For this review, take the finished solid that the model builds, in its own axes (mm). A direction names the side the tool comes from. Round coordinates to 2 decimals unless told otherwise and drop trailing zeros. Order: outer loops, then holes, each group sorted by start corner. A loop starts at its lowest first (then second) coordinate and runs counter-clockwise, first axis right, second up. Notation, with made-up numbers: M 11,32.5 L 42,32.5 A23 cw 42,56.5 Z; hole C 80.25,77 d6. An arc over 180 degrees is marked long. Use a Markdown table: item, result.
from build123d import *

# Parameters (mm, degrees)
SKETCH2_W            = 59
SKETCH2_H            = 39.64
BOSS_EXTRUDE1_DEPTH  = 2
BOSS_EXTRUDE2_DEPTH  = 87.25
SKETCH4_W            = 59
SKETCH4_H            = 39.64
BOSS_EXTRUDE4_DEPTH  = 2
BOSS_EXTRUDE5_DEPTH  = 59
SKETCH5_3_W          = 2
SKETCH5_3_H          = 10
BOSS_EXTRUDE6_DEPTH  = 59
BOSS_EXTRUDE7_DEPTH  = 59
BOSS_EXTRUDE8_DEPTH  = 6
SKETCH8_W            = 38.6
SKETCH8_H            = 87.25
CUT_EXTRUDE1_DEPTH   = 12.5
SKETCH9_W            = 15.5
SKETCH9_H            = 10.65
CUT_EXTRUDE2_DEPTH   = 13.6
SKETCH9_4_W          = 21.1
SKETCH9_4_H          = 7.5
CUT_EXTRUDE3_DEPTH   = 8.6
SKETCH10_W           = 67.65
SKETCH10_H           = 14.625
BOSS_EXTRUDE9_DEPTH  = 7.9
BOSS_EXTRUDE10_DEPTH = 4
SKETCH11_W           = 25
SKETCH11_H           = 7.9
BOSS_EXTRUDE14_DEPTH = 22
SKETCH12_W           = 25
SKETCH12_H           = 10
CUT_EXTRUDE4_DEPTH   = 3.9


with BuildPart() as part:
    # Sketch2 → Boss-Extrude1 (new body)
    with BuildSketch(Plane.XY):
        Polygon((-256.9, 47.64), (-256.9, 0), (0, 0), (0, 41.64), (-2, 41.64), (-2, 9.9), (-8.85, 9.9), (-8.85, 2), (-144.15, 2), (-144.15, 9.9), (-151, 9.9), (-151, 41.64), (-153, 41.64), (-191.6, 41.64), (-193.6, 41.64), (-193.6, 2), (-252.6, 2), (-252.6, 41.64), (-254.9, 41.64), (-254.9, 45.64), (-252.6, 45.64), (-252.6, 47.64), align=None)
        with Locations((-223.1, 21.82)):
            Rectangle(SKETCH2_W, SKETCH2_H)
        Polygon((-151, 41.64), (-2, 41.64), (-2, 9.9), (-8.85, 9.9), (-8.85, 2), (-144.15, 2), (-144.15, 9.9), (-151, 9.9), align=None)
    extrude(amount=-BOSS_EXTRUDE1_DEPTH)

    # Sketch2_3 → Boss-Extrude2 (add)
    with BuildSketch(Plane.XY):
        Polygon((-256.9, 47.64), (-256.9, 0), (0, 0), (0, 41.64), (-2, 41.64), (-2, 9.9), (-8.85, 9.9), (-8.85, 2), (-144.15, 2), (-144.15, 9.9), (-151, 9.9), (-151, 41.64), (-153, 41.64), (-191.6, 41.64), (-193.6, 41.64), (-193.6, 2), (-252.6, 2), (-252.6, 41.64), (-254.9, 41.64), (-254.9, 45.64), (-252.6, 45.64), (-252.6, 47.64), align=None)
    extrude(amount=BOSS_EXTRUDE2_DEPTH)

    # Sketch4 → Boss-Extrude4 (add)
    with BuildSketch(Plane.XY.offset(87.25)):
        Polygon((-256.9, 47.64), (-256.9, 41.64), (-254.9, 41.64), (-254.9, 45.64), (-252.6, 45.64), (-252.6, 47.64), align=None)
        with Locations((-223.1, 21.82)):
            Rectangle(SKETCH4_W, SKETCH4_H)
        Polygon((-254.9, 41.64), (-256.9, 41.64), (-256.9, 0), (0, 0), (0, 41.64), (-2, 41.64), (-2, 9.9), (-8.85, 9.9), (-8.85, 2), (-144.15, 2), (-144.15, 9.9), (-151, 9.9), (-151, 41.64), (-193.6, 41.64), (-193.6, 2), (-252.6, 2), (-252.6, 41.64), align=None)
        Polygon((-2, 41.64), (-151, 41.64), (-151, 9.9), (-144.15, 9.9), (-144.15, 2), (-8.85, 2), (-8.85, 9.9), (-2, 9.9), align=None)
    extrude(amount=BOSS_EXTRUDE4_DEPTH)

    # Sketch5 → Boss-Extrude5 (add)
    with BuildSketch(Plane(origin=(-252.6, 0, 0), x_dir=(0, 0, -1), z_dir=(1, 0, 0))):
        Polygon((-72.69, 2), (-40.014243309, 31.64), (-42.014243309, 31.64), (-56.208170838, 18.764766047), (-87.25, 18.764766047), (-87.25, 2), align=None)
        Polygon((0, 2), (0, 31.64), (-10, 31.64), (-21.014243309, 31.64), (-53.69, 2), align=None)
    extrude(amount=BOSS_EXTRUDE5_DEPTH)

    # Sketch5_3 → Boss-Extrude6 (add)
    with BuildSketch(Plane(origin=(-252.6, 0, 0), x_dir=(0, 0, -1), z_dir=(1, 0, 0))):
        with Locations((-41.014243309, 36.64)):
            Rectangle(SKETCH5_3_W, SKETCH5_3_H)
    extrude(amount=BOSS_EXTRUDE6_DEPTH)

    # Sketch6 → Boss-Extrude7 (add)
    with BuildSketch(Plane(origin=(-252.6, 0, 0), x_dir=(0, 0, -1), z_dir=(1, 0, 0))):
        with BuildLine():
            Line((-42.014243309, 31.64), (-42.014243309, 41.64))
            ThreePointArc((-42.014243309, 41.64), (-48.969941413, 25.441110515), (-65.285951379, 18.764766047))
            Line((-65.285951379, 18.764766047), (-56.208170838, 18.764766047))
            Line((-56.208170838, 18.764766047), (-42.014243309, 31.64))
        make_face()
    extrude(amount=BOSS_EXTRUDE7_DEPTH)

    # Sketch7 → Boss-Extrude8 (add)
    with BuildSketch(Plane(origin=(0, 41.64, 0), x_dir=(1, 0, 0), z_dir=(0, 1, 0))):
        Polygon((0, -89.25), (0, 2), (-254.9, 2), (-254.9, 0), (-252.6, 0), (-2, 0), (-2, -87.25), (-252.6, -87.25), (-254.9, -87.25), (-254.9, -89.25), align=None)
    extrude(amount=BOSS_EXTRUDE8_DEPTH)

    # Sketch8 → Cut-Extrude1 (cut)
    with BuildSketch(Plane(origin=(0, 41.64, 0), x_dir=(1, 0, 0), z_dir=(0, 1, 0))):
        with Locations((-172.3, -43.625)):
            Rectangle(SKETCH8_W, SKETCH8_H)
    extrude(amount=-CUT_EXTRUDE1_DEPTH, mode=Mode.SUBTRACT)

    # Sketch9 → Cut-Extrude2 (cut)
    with BuildSketch(Plane(origin=(0, 29.14, 0), x_dir=(1, 0, 0), z_dir=(0, 1, 0))):
        with Locations((-160.75, -16.325)):
            Rectangle(SKETCH9_W, SKETCH9_H)
        with Locations((-183.85, -29.975)):
            Rectangle(SKETCH9_W, SKETCH9_H)
        with Locations((-160.75, -43.625)):
            Rectangle(SKETCH9_W, SKETCH9_H)
        with Locations((-183.85, -57.275)):
            Rectangle(SKETCH9_W, SKETCH9_H)
        with Locations((-160.75, -70.925)):
            Rectangle(SKETCH9_W, SKETCH9_H)
    extrude(amount=-CUT_EXTRUDE2_DEPTH, mode=Mode.SUBTRACT)

    # Sketch9_4 → Cut-Extrude3 (cut)
    with BuildSketch(Plane(origin=(0, 29.14, 0), x_dir=(1, 0, 0), z_dir=(0, 1, 0))):
        with Locations((-181.05, -16.325)):
            Rectangle(SKETCH9_4_W, SKETCH9_4_H)
        with Locations((-163.55, -29.975)):
            Rectangle(SKETCH9_4_W, SKETCH9_4_H)
        with Locations((-181.05, -43.625)):
            Rectangle(SKETCH9_4_W, SKETCH9_4_H)
        with Locations((-163.55, -57.275)):
            Rectangle(SKETCH9_4_W, SKETCH9_4_H)
        with Locations((-181.05, -70.925)):
            Rectangle(SKETCH9_4_W, SKETCH9_4_H)
    extrude(amount=-CUT_EXTRUDE3_DEPTH, mode=Mode.SUBTRACT)

    # Sketch10 → Boss-Extrude9 (add)
    with BuildSketch(Plane(origin=(0, 2, 0), x_dir=(1, 0, 0), z_dir=(0, 1, 0))):
        with Locations((-110.325, -7.3125)):
            Rectangle(SKETCH10_W, SKETCH10_H)
        with Locations((-42.675, -7.3125)):
            Rectangle(SKETCH10_W, SKETCH10_H)
        with Locations((-42.675, -79.9375)):
            Rectangle(SKETCH10_W, SKETCH10_H)
        with Locations((-110.325, -79.9375)):
            Rectangle(SKETCH10_W, SKETCH10_H)
    extrude(amount=BOSS_EXTRUDE9_DEPTH)

    # Sketch10_4 → Boss-Extrude10 (add)
    with BuildSketch(Plane(origin=(0, 2, 0), x_dir=(1, 0, 0), z_dir=(0, 1, 0))):
        Polygon((-8.85, -36.625), (-144.15, -36.625), (-144.15, -72.625), (-76.5, -72.625), (-8.85, -72.625), align=None)
    extrude(amount=BOSS_EXTRUDE10_DEPTH)

    # Sketch11 → Boss-Extrude14 (add)
    with BuildSketch(Plane.XY.offset(14.625)):
        with Locations((-131.65, 5.95)):
            Rectangle(SKETCH11_W, SKETCH11_H)
        with Locations((-21.35, 5.95)):
            Rectangle(SKETCH11_W, SKETCH11_H)
    extrude(amount=BOSS_EXTRUDE14_DEPTH)

    # Sketch12 → Cut-Extrude4 (cut)
    with BuildSketch(Plane(origin=(0, 9.9, 0), x_dir=(1, 0, 0), z_dir=(0, 1, 0))):
        with Locations((-131.65, -31.625)):
            Rectangle(SKETCH12_W, SKETCH12_H)
        with Locations((-21.35, -31.625)):
            Rectangle(SKETCH12_W, SKETCH12_H)
    extrude(amount=-CUT_EXTRUDE4_DEPTH, mode=Mode.SUBTRACT)


solid = part.part
Q1. Add section C-C (y = 38). Write out the cut boundary in (x, z).
Determined:
| item | result |
|---|---|
| outline | M -256.9,-2 L 0,-2 L 0,89.25 L -256.9,89.25 Z; hole M -252.6,0 L -193.6,0 L -193.6,40.01 L -252.6,40.01 Z; hole M -252.6,42.36 L -193.6,42.36 L -193.6,87.25 L -252.6,87.25 Z; hole M -191.6,0 L -153,0 L -153,87.25 L -191.6,87.25 Z; hole M -151,0 L -2,0 L -2,87.25 L -151,87.25 Z |
Q2. Wall thickness on line 1 along X through (y, z) = (31, 25.5); line 2 along Z through (x, y) = (-172, 26) (3 decimals); line 3 along X through (y, z) = (9, 49.5): over which ranges is each line inside the solid? List them lowest first. Write a range as [from, to].
Determined:
| item | result |
|---|---|
| line 1 | x = [-256.9, -252.6], [-193.6, -191.6], [-153, -151], [-2, 0] |
| line 2 | z = [-2, 12.575], [20.075, 26.225], [33.725, 39.875], [47.375, 53.525], [61.025, 67.175], [74.675, 89.25] |
| line 3 | x = [-256.9, -252.6], [-193.6, -144.15], [-8.85, 0] |
Q3. Machinability: for faces 4 (the flat face through (-164, 20.54, 30)), 5 (the flat face through (-223, 2, 63)), which of the approach directions +Z, -Z, +X, -X, +Y, -Y give a long, thin tool a straight path to every point of the face, cutting with its end or side? Answer none if there is none.
Determined:
| item | result |
|---|---|
| face 4 | +Y |
| face 5 | none |
Q4. Add section A-A (x = -208.5). Write out the cut boundary in (y, z), then the cut area to 3 significant figures.
Determined:
| item | result |
|---|---|
| outline | M 0,-2 L 47.64,-2 L 47.64,0 L 31.64,0 L 31.64,21.01 L 2,53.69 L 2,72.69 L 31.64,40.01 L 41.64,40.01 L 41.64,42.01 A23.28 cw 18.76,65.29 L 18.76,87.25 L 47.64,87.25 L 47.64,89.25 L 0,89.25 Z |
| area | 1,940 mm^2 |
Q5. Clearance check with flat-ended pins moving along their axes: pin 1 (8 mm diameter, centred on x = -178, z = 72, fed in from +Y); pin 2 (3 mm diameter, centred on x = -124.5, z = 66, fed in from +Y); pin 3 (2 mm diameter, centred on x = -151.5, z = 24, fed in from +Y). State where each tip first meets the part, or that it passes through.
Determined:
| item | result |
|---|---|
| pin 1 | stops at y = 29.14 |
| pin 2 | stops at y = 6 |
| pin 3 | stops at y = 41.64 |
Q6. Add section B-B (z = 5.5). Write out the cut boundary in (x, y).
Determined:
| item | result |
|---|---|
| outline | M -256.9,0 L 0,0 L 0,47.64 L -2,47.64 L -2,9.9 L -151,9.9 L -151,41.64 L -153,41.64 L -153,29.14 L -191.6,29.14 L -191.6,41.64 L -193.6,41.64 L -193.6,31.64 L -252.6,31.64 L -252.6,41.64 L -254.9,41.64 L -254.9,45.64 L -252.6,45.64 L -252.6,47.64 L -256.9,47.64 Z |
Q7. Draft analysis for pull direction X (two halves, no side actions). For faces 1 (the flat face through (-252.6, 25, 36)), 2 (the flat face through (0, 23, 44)), 3 (the flat face through (-127, 23, -2)), state which applies: pulls with the +X half, pulls with the -X half, needs draft (parallel to the pull), parting line crosses it, or undercut.
Determined:
| item | result |
|---|---|
| face 1 | undercut |
| face 2 | pulls with the +X half |
| face 3 | needs draft |
Q8. Add section D-D (z = 82.5). Write out the cut boundary in (x, y).
Determined:
| item | result |
|---|---|
| outline | M -256.9,0 L 0,0 L 0,47.64 L -2,47.64 L -2,9.9 L -151,9.9 L -151,41.64 L -153,41.64 L -153,29.14 L -191.6,29.14 L -191.6,41.64 L -193.6,41.64 L -193.6,18.76 L -252.6,18.76 L -252.6,41.64 L -254.9,41.64 L -254.9,45.64 L -252.6,45.64 L -252.6,47.64 L -256.9,47.64 Z |
